Autodesk Inventor part; units mm, degrees
ref_plane "YZ Plane" through (0, 0, 0) normal (1, 0, 0) x (0, 1, 0)
ref_plane "XZ Plane" through (0, 0, 0) normal (0, 1, 0) x (-1, 0, 0)
ref_plane "XY Plane" through (0, 0, 0) normal (0, 0, 1) x (1, 0, 0)
sketch "Sketch1" plane through (0, 0, 0) normal (0, 1, 0) x (-1, 0, 0)
  circle A0 centre (0, 0) radius 2
  dimension "d0" = 4
extrude "Extrusion1" add sketch "Sketch1" against normal blind 80
sketch "Sketch2" plane through (0, -80, 0) normal (0, -1, 0) x (1, 0, 0)
  circle A0 centre (0, 0) radius 2
  line L0 (-1.3229, 1.5) -> (1.3229, 1.5)
  circle A1 centre (0, 0) radius 2
  dimension "d3" = 0.5
extrude "Extrusion2" cut sketch "Sketch2" against normal through all contours L0 A0 picked at (-0.3089, 1.5908)
chamfer "Chamfer1" distance 0.2 angle 45 4 edges at (0, -80, -2) (0, -80, 1.5) (0, 0, -2) (0, 0, 1.5)
properties part number "10-0080" material "Aluminum 6061"
Geometry: final body of the model. Coordinates: model frame, mm. Coordinates: 2 decimals unless noted, no trailing zeros. Order: outer loops, then holes, each group sorted by start corner. A loop starts at its lowest first (then second) coordinate and runs counter-clockwise, first axis right, second up. Notation, with made-up numbers: (64, 83) -> (83, 83) arc R13 ccw to (83, 99) -> close; hole circle Ø6 at (0, 88.25). An arc over 180 degrees is marked (long way). Write item = value, one per line.
(1) Line query: line 1 (Z direction, x = -1.5, y = -11); line 2 (Z direction, x = -0.25, y = -20.5); line 3 (X direction, y = -26, z = -0.1). Output: solid intervals per line, ascending.
Solved:
line_1 = -1.32 to 1.32
line_2 = -1.98 to 1.5
line_3 = -2 to 2
(2) Pin query (flat end, axial travel): pin 1 Ø1 at (x, y) = (-1.5, -21.5) entering from -Z. Return the tip coordinate at first contact, or that it passes through.
Solved:
pin_1 = -1.73
(3) Cut plane A-A on y = -70.5. Return loops of the section in (x, z), plus the area to 3 significant figures.
Solved:
outline = (-1.32, 1.5) arc R2 ccw (long way) to (1.32, 1.5) -> close
area = 11.7 mm²
